Could you check a few things on this model? Use its own coordinates, in mm. Give positions to 0.01 mm unless a question says otherwise; leave off trailing zeros. Order: outer loops, then holes, each group sorted by start corner. A loop starts at its lowest first (then second) coordinate and runs counter-clockwise, first axis right, second up. Notation, with made-up numbers: (-19, -39.5) - (29, -39.5) arc R15 ccw to (29, -23.5) - close; hole circle Ø4 at (37, 88). An arc over 180 degrees is marked (long way). One line per question, with ' | ' between items. Start each with the question number.
1. For P1, Ø1.5, axis at x = 327.5, y = 0.5, coming from the -Z side; P2, Ø5, axis at x = 66.5, y = 1, coming from the +Z side; P3, Ø5, axis at x = 84.5, z = 7.5, coming from the -Y side, each with a flat end and sliding along its axis, tell me the tip position at first contact or that it passes through.
2. If we mould it in two halves opening along Z, with no side actions, what happens to faces 1 (the cylindrical face through (187.833, -15.517, -11.898)), 2 (the flat face through (381, -9, -4)), 3 (the cylindrical face through (187.833, 7.559, -5.796))? For each: released by +Z, released by -Z, zero draft, split by the parting line, or undercut.
3. Imagine slicing it at D-D (y = -16). Please give me the cut outline in (x, z).
4. Imagine slicing it at C-C (x = 76). Please give me the cut outline in (y, z) (3 decimals), and give its area (3 significant figures).
5. Imagine slicing it at A-A (z = 0). Please give me the cut outline in (x, y) (3 decimals), and give its area (3 significant figures).
6. I need wall thicknesses on probe 1 along Z at (x, y) = (270.5, 1); probe 2 along Z at (x, y) = (250, 0) (3 decimals); probe 3 along Y at (x, z) = (110, 0.5). Which ranges of each line are inside material? Lowest first, please. Write a range as from..to.
```python
from build123d import *

# Parameters (mm, degrees)
F0_R     = 19.5535243405
F1_DEPTH = 127
F3_D     = 19.05
F4_DEPTH = 254


with BuildPart() as f1:
    # F0 (on Right) → F1 (new body)
    with BuildSketch(Plane.YZ):
        Circle(F0_R)
    extrude(amount=F1_DEPTH)

    # F3 (through all)
    with Locations(Plane.YZ.offset(127)):
        with Locations((0, 0)):
            Hole(F3_D / 2)

    # F4 (add): a face of the model
    f4_faces = [f1.faces().sort_by_distance(p)[0] for p in [
        (127, -19.0004671542, 0),
    ]]
    extrude(f4_faces, amount=F4_DEPTH)


solid = f1.part
```
Results found:
1) P1: stops at z = -19.55 | P2: stops at z = 19.55 | P3: stops at y = -18.9
2) face 1: split by the parting line | face 2: zero draft | face 3: undercut
3) outline: (0, -11.24) - (381, -11.24) - (381, 11.24) - (0, 11.24) - close
4) outline: circle Ø39.107 at (0, 0); hole circle Ø19.05 at (0, 0) | area: 916 mm2
5) outline: (0, -19.554) - (381, -19.554) - (381, -9.525) - (0, -9.525) - close; (0, 9.525) - (381, 9.525) - (381, 19.554) - (0, 19.554) - close | area: 7,640 mm2
6) probe 1: z = -19.53..-9.47, 9.47..19.53 | probe 2: z = -19.554..-9.525, 9.525..19.554 | probe 3: y = -19.55..-9.51, 9.51..19.55
